Verification items for this drawing (mm, ordinates from the low corner). A direction names the side the tool comes from. Coordinates: 2 decimals unless noted, no trailing zeros. Order: outer loops, then holes, each group sorted by start corner. A loop starts at its lowest first (then second) coordinate and runs counter-clockwise, first axis right, second up. Notation, with made-up numbers: M -11.5,-29 L -7.5,-29 A15 cw -7.5,-7 Z; hole C 76,39.5 d10. An arc over 180 degrees is marked long. Return JSON: item names as keys, results as strings. Group by question number.
1. Mould release check, pull along Y, two halves, no side actions. Record for the marked faces 4, 5 and 6: +Y half, -Y half, draft (parallel to the pull), parting line (faces both ways), or undercut.
2. Material ranges on line 1 along Z through (x, y) = (12, 13.25); line 2 along X through (y, z) = (8.15, 2.56); line 3 along Y through (x, z) = (15.75, 3.8), recorded low to high.
3. Section check B-B, the plane z = 2.56. Record the cut outline in (x, y), plus the area to 3 significant figures.
4. Set-up check for the marked faces 1, 2 and 3: record each of +Z, -Z, +X, -X, +Y, -Y from which the full face is reachable in a straight line by a thin tool's end or side.
5. Section check A-A, the plane y = 7.5. Record the cut outline in (x, z) (3 decimals).
6. Gauge pin test, flat ends, axial feed: pin 1 (2.5 mm diameter, centred on x = 15.5, z = 2, fed in from -Y); pin 2 (8 mm diameter, centred on x = 6.33, y = 7.5, fed in from +Z); pin 3 (2 mm diameter, centred on x = 7, z = 1.5, fed in from +Y); pin 4 (2 mm diameter, centred on y = 7.5, z = 2, fed in from -X). Record the tip position at first contact, or that the pin passes through.
7. Section check D-D, the plane y = 9. Record the cut outline in (x, z) (3 decimals).
8. Section check C-C, the plane x = 7.25. Record the cut outline in (y, z), plus the area to 3 significant figures.
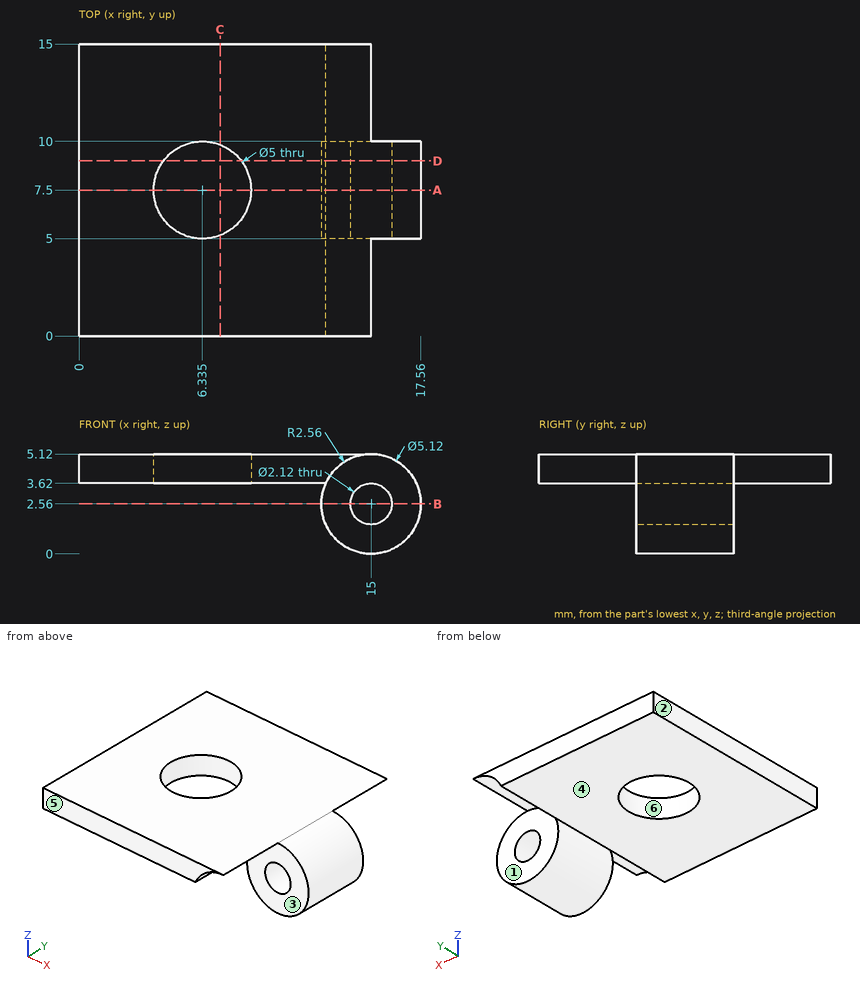
Answers follow:
{
 "1": {"face 4": "draft", "face 5": "-Y half", "face 6": "undercut"},
 "2": {"line 1": "3.62 to 5.12", "line 2": "12.44 to 13.94, 16.06 to 17.56", "line 3": "5 to 10"},
 "3": {"outline": "M 12.44,5 L 13.94,5 L 13.94,10 L 12.44,10 Z; M 16.06,5 L 17.56,5 L 17.56,10 L 16.06,10 Z", "area": "15.0 mm^2"},
 "4": {"face 1": "-Z, +X, +Y", "face 2": "+Z, -Z, -X, +Y, -Y", "face 3": "-Z, +X, -Y"},
 "5": {"outline": "M 0,3.62 L 3.835,3.62 L 3.835,5.12 L 0,5.12 Z; M 8.835,3.62 L 12.67,3.62 A2.56 ccw long 15,5.12 L 8.835,5.12 Z; hole C 15,2.56 d2.12"},
 "6": {"pin 1": "y = 5", "pin 2": "z = 5.12", "pin 3": "through", "pin 4": "x = 12.44"},
 "7": {"outline": "M 0,3.62 L 4.335,3.62 L 4.335,5.12 L 0,5.12 Z; M 8.335,3.62 L 12.67,3.62 A2.56 ccw long 15,5.12 L 8.335,5.12 Z; hole C 15,2.56 d2.12"},
 "8": {"outline": "M 0,3.62 L 5.17,3.62 L 5.17,5.12 L 0,5.12 Z; M 9.83,3.62 L 15,3.62 L 15,5.12 L 9.83,5.12 Z", "area": "15.5 mm^2"}
}
